from build123d import *

# Parameters (mm, degrees)
SKETCH1_R           = 6
SKETCH1_R_2         = 5
BOSS_EXTRUDE1_DEPTH = 15


with BuildPart() as part:
    # Sketch1 → Boss-Extrude1 (new body)
    with BuildSketch(Plane.XY):
        with BuildLine():
            Line((-80, 30), (-40, 30))
            Line((-40, 30), (4.685564793, 11.047419724))
            ThreePointArc((4.685564793, 11.047419724), (12, 0), (4.685564793, -11.047419724))
            Line((4.685564793, -11.047419724), (-40, -30))
            Line((-40, -30), (-80, -30))
            Line((-80, -30), (-80, -10))
            Line((-80, -10), (-60, -10))
            ThreePointArc((-60, -10), (-50, 0), (-60, 10))
            Line((-60, 10), (-80, 10))
            Line((-80, 10), (-80, 30))
        make_face()
        Circle(SKETCH1_R, mode=Mode.SUBTRACT)
        with Locations((-70, 20)):
            Circle(SKETCH1_R_2, mode=Mode.SUBTRACT)
        with Locations((-50, 20)):
            Circle(SKETCH1_R_2, mode=Mode.SUBTRACT)
        with Locations(Location((-70, -20, 0), (0, 0, 180))):
            Circle(SKETCH1_R_2, mode=Mode.SUBTRACT)
        with Locations(Location((-50, -20, 0), (0, 0, 180))):
            Circle(SKETCH1_R_2, mode=Mode.SUBTRACT)
    extrude(amount=BOSS_EXTRUDE1_DEPTH)


solid = part.part
Check sheet for the modelled part. Datum: model origin and axes. Units: mm. A direction names the side the tool comes from. Round coordinates to 2 decimals unless told otherwise and drop trailing zeros. Order: outer loops, then holes, each group sorted by start corner. A loop starts at its lowest first (then second) coordinate and runs counter-clockwise, first axis right, second up.
Q1. Cross-section at C-C, the plane z = 13.5. Enter the section's corners in (x, y).
Filled sheet:
outline: (-80, -30) - (-40, -30) - (4.69, -11.05) arc R12 ccw to (4.69, 11.05) - (-40, 30) - (-80, 30) - (-80, 10) - (-60, 10) arc R10 cw to (-60, -10) - (-80, -10) - close; hole circle Ø10 at (-70, -20); hole circle Ø10 at (-70, 20); hole circle Ø10 at (-50, -20); hole circle Ø10 at (-50, 20); hole circle Ø12 at (0, 0)
Q2. Draft check along X on faces 3 (the face through (-70, 10, 7)), 4 (the face through (-65.381, 18.085, 7.395)), 5 (the face through (12, 0, 7)), 6 (the face through (-80, -20, 7)). Enter one of: pulls with the +X half, pulls with the -X half, needs draft (parallel to the pull), parting line crosses it, or undercut.
Filled sheet:
face 3: needs draft
face 4: undercut
face 5: pulls with the +X half
face 6: pulls with the -X half
Q3. Cross-section at B-B, the plane x = -70. Enter the section's corners in (y, z).
Filled sheet:
outline: (-30, 0) - (-25, 0) - (-25, 15) - (-30, 15) - close; (-15, 0) - (-10, 0) - (-10, 15) - (-15, 15) - close; (10, 0) - (15, 0) - (15, 15) - (10, 15) - close; (25, 0) - (30, 0) - (30, 15) - (25, 15) - close
Q4. Scan lines: L1, parallel to X at y = -20, z = 14; L2, parallel to Y at x = -68, z = 5.5; L3, parallel to X at y = 16.5, z = 2.75. Record each from-to range of solid material in increasing order.
Filled sheet:
L1: x = -80 to -75, -65 to -55, -45 to -16.42
L2: y = -30 to -24.58, -15.42 to -10, 10 to 15.42, 24.58 to 30
L3: x = -80 to -73.57, -66.43 to -53.57, -46.43 to -8.17
Q5. Cross-section at A-A, the plane y = 0. Enter the section's corners in (x, z), plus the area to 3 significant figures.
Filled sheet:
outline: (-50, 0) - (-6, 0) - (-6, 15) - (-50, 15) - close; (6, 0) - (12, 0) - (12, 15) - (6, 15) - close
area: 750 mm2
Q6. Depth check by flat-ended pin: P1, Ø16, axis at x = -50, y = -20, coming from the +Z side; P2, Ø3, axis at x = -37, z = 2.5, coming from the -Y side; P3, Ø1, axis at x = -3.5, z = 10.5, coming from the +Y side; P4, Ø3, axis at x = 2.5, z = 3.5, coming from the -Y side. Enter the tip coordinate at first touch or a pass-through.
Filled sheet:
P1: stops at z = 15
P2: stops at y = -29.36
P3: stops at y = 14.73
P4: stops at y = -12.61
Q7. Set-up check for faces 1 (the face through (-74.619, -18.085, 7.395)), 2 (the face through (-70, -10, 7)): record each of +Z, -Z, +X, -X, +Y, -Y from which the full face is reachable in a straight line by a thin tool's end or side.
Filled sheet:
face 1: +Z, -Z
face 2: +Z, -Z, -X
Q8. Cross-section at D-D, the plane x = 0. Enter the section's corners in (y, z).
Filled sheet:
outline: (-13.03, 0) - (-6, 0) - (-6, 15) - (-13.03, 15) - close; (6, 0) - (13.03, 0) - (13.03, 15) - (6, 15) - close
